Build history of the part. All positions in model axes, mm. A direction names the side the tool comes from. Give positions to 0.01 mm unless a question says otherwise; leave off trailing zeros. Loops run counter-clockwise (first coordinate to the right, second up) from the corner with the lowest first, then second, coordinate; pieces in that order, holes last. Notation, with made-up numbers: (68.25, 3) - (86.25, 3) arc R16 cw to (86.25, 25) - close; hole circle Ø2 at (73, 64.25). An arc over 180 degrees is marked (long way). Return JSON: item names as keys, results as strings. Group by question number.
1) Drop flat-ended pins along their axis: pin 1 (5.5 mm diameter, centred on x = -10, z = -2, fed in from -Y); pin 2 (1.5 mm diameter, centred on x = -67.5, y = 2.5, fed in from -Z); pin 3 (1 mm diameter, centred on y = 3, z = -7.5, fed in from +X). Give the stop position or say it passes through.
2) Mould opens along Z. For faces 3 (the face through (-12.4, 2, -3.8)), 4 (the face through (-44, 4, -5)), 5 (the face through (-88, 2, -5)), 6 (the face through (-68.863, 1.972, 1.275)) say: released by +Z, released by -Z, zero draft, split by the parting line, or undercut.
3) Slice it at A-A (y = 3). List the corners of the cut face in (x, z).
4) 3-axis set-ups, long thin cutter, end or side, ignore diameter. For faces 1 (the face through (-102.52, 1.97, 1.62)), 2 (the face through (-44, 0, -5)): which of +Z, -Z, +X, -X, +Y, -Y reach the whole face in a straight line?
5) Slice it at B-B (x = -94). List the corners of the cut face in (y, z), and give its area (3 significant figures).
6) Drill centre lines: probe 1 along Z at (x, y) = (-10, 2); probe 2 along Z at (x, y) = (-85, 1); probe 3 along Z at (x, y) = (-95, 2.35). Where is each one in solid material? Low to high. Write a range as from..to.
7) Slice it at C-C (x = -70). List the corners of the cut face in (y, z), and give its area (3 significant figures).
Autodesk Inventor part; units mm, degrees
ref_plane "YZ Plane" through (0, 0, 0) normal (1, 0, 0) x (0, 1, 0)
ref_plane "XZ Plane" through (0, 0, 0) normal (0, 1, 0) x (-1, 0, 0)
ref_plane "XY Plane" through (0, 0, 0) normal (0, 0, 1) x (1, 0, 0)
sketch "スケッチ1" plane through (0, 0, 0) normal (0, 1, 0) x (-1, 0, 0)
  arc A0 (120.7701, -0.6068) -> (119.8564, 3.2634) centre (120.103, 1.2786) ccw
  arc A1 (41.4452, -14.9694) -> (120.7701, -0.6068) centre (36.8758, 236.5065) ccw
  arc A2 (30.7183, -14.8468) -> (41.4452, -14.9694) centre (38.1525, 166.2425) ccw
  arc A3 (11.0166, -11.3447) -> (30.7183, -14.8468) centre (33.77, 59.49) ccw
  arc A4 (-0.3565, -5.7585) -> (11.0166, -11.3447) centre (24.3575, 30.1875) ccw
  arc A5 (-3.5852, -2.6234) -> (-0.3565, -5.7585) centre (7.25, 5.305) ccw
  arc A6 (-0.7848, 4.3726) -> (-3.5852, -2.6234) centre (0, 0) ccw
  arc A7 (7.6183, 5.1344) -> (-0.7848, 4.3726) centre (7.775, -43.32) ccw
  arc A8 (35.5607, 3.8888) -> (7.6183, 5.1344) centre (8.565, -287.665) ccw
  arc A9 (35.5607, 3.8888) -> (52.6853, 2.3311) centre (526.9475, 5310.875) ccw
  arc A10 (52.6853, 2.3311) -> (84.6244, 0.9905) centre (82.86, 340.0849) ccw
  arc A11 (84.6244, 0.9905) -> (119.8564, 3.2634) centre (83.0725, 299.245) ccw
extrude "押し出し1" add sketch "スケッチ1" along normal blind 4
sketch "スケッチ2" plane through (0, 0, 0) normal (0, -1, 0) x (1, 0, 0)
  circle A0 centre (-10, -2) radius 3
  circle A1 centre (-85, -5) radius 3
  point P0 (0, 0)
  dimension "d3" = 6
  dimension "d4" = 6
  dimension "d5" = 10
  dimension "d6" = 2
  dimension "d7" = 5
  dimension "d8" = 85
extrude "押し出し2" cut sketch "スケッチ2" against normal through all
equation "\"d4\" = d3"
properties part number "plate_sf2" material "木材 (オーク)"
Results:
{
 "1": {"pin 1": "through", "pin 2": "z = -13.23", "pin 3": "x = -1.55"},
 "2": {"face 3": "undercut", "face 4": "zero draft", "face 5": "undercut", "face 6": "released by +Z"},
 "3": {"outline": "(-120.77, -0.61) arc R251.51 ccw to (-41.45, -14.97) arc R181.22 ccw to (-30.72, -14.85) arc R74.4 ccw to (-11.02, -11.34) arc R43.63 ccw to (0.36, -5.76) arc R13.42 ccw to (3.59, -2.62) arc R4.44 ccw to (0.78, 4.37) arc R48.46 ccw to (-7.62, 5.13) arc R292.8 ccw to (-35.56, 3.89) arc R5310.23 cw to (-52.69, 2.33) arc R339.09 cw to (-84.62, 0.99) arc R298.26 cw to (-119.86, 3.26) arc R2 ccw to start; hole circle Ø6 at (-85, -5); hole circle Ø6 at (-10, -2)"},
 "4": {"face 1": "+Z, +Y, -Y", "face 2": "+Z, -Z, +X, -X, -Y"},
 "5": {"outline": "(0, -8.44) - (4, -8.44) - (4, 1.19) - (0, 1.19) - close", "area": "38.5 mm2"},
 "6": {"probe 1": "-11..-5, 1..5.13", "probe 2": "-10.36..-8, -2..0.99", "probe 3": "-8.2..1.23"},
 "7": {"outline": "(0, -12.82) - (4, -12.82) - (4, 1.23) - (0, 1.23) - close", "area": "56.2 mm2"}
}
